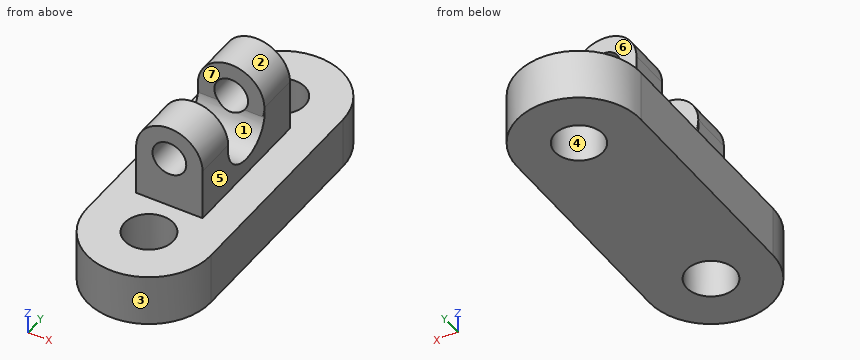
from build123d import *

# Parameters (mm, degrees)
F0_W      = 32.9013951123
F0_H      = 70.9037855268
F1_DEPTH  = 25.4
F2_DEPTH  = 50.8
F3_R      = 14.9412695824
F4_DEPTH  = 76.2
F5_W      = 16.4506975561
F5_H      = 20.7484884761
F7_W      = 16.4506975561
F7_H      = 20.7484884761
F9_R      = 8.3599226064
F10_DEPTH = 508


with BuildPart() as f1:
    # F0 (on Top) → F1 (new body)
    with BuildSketch(Plane.XY):
        with BuildLine():
            Line((28.4018162638, 52.9936365783), (9.7189312353, 52.9936365783))
            ThreePointArc((9.7189312353, 52.9936365783), (-2.1936381236, 41.0810672195), (-14.1062074824, 52.9936365783))
            Line((-14.1062074824, 52.9936365783), (-32.7890925109, 52.9936365783))
            Line((-32.7890925109, 52.9936365783), (-32.7890925109, -54.1481785476))
            Line((-32.7890925109, -54.1481785476), (-14.2189597558, -54.1481785476))
            ThreePointArc((-14.2189597558, -54.1481785476), (-2.1936381236, -42.1228569154), (9.8316835087, -54.1481785476))
            Line((9.8316835087, -54.1481785476), (28.4018162638, -54.1481785476))
            Line((28.4018162638, -54.1481785476), (28.4018162638, 52.9936365783))
        make_face()
        with Locations((-4.080792889, 0.9530261159)):
            Rectangle(F0_W, F0_H, mode=Mode.SUBTRACT)
        with BuildLine():
            ThreePointArc((-14.1062074824, 52.9936365783), (-2.1936381236, 64.9062059372), (9.7189312353, 52.9936365783))
            Line((9.7189312353, 52.9936365783), (28.4018162638, 52.9936365783))
            ThreePointArc((28.4018162638, 52.9936365783), (-2.1936381236, 83.5890909657), (-32.7890925109, 52.9936365783))
            Line((-32.7890925109, 52.9936365783), (-14.1062074824, 52.9936365783))
        make_face()
        with BuildLine():
            ThreePointArc((-32.7890925109, -54.1481785476), (-2.1936381236, -84.743632935), (28.4018162638, -54.1481785476))
            Line((28.4018162638, -54.1481785476), (9.8316835087, -54.1481785476))
            ThreePointArc((9.8316835087, -54.1481785476), (-2.1936381236, -66.1735001799), (-14.2189597558, -54.1481785476))
            Line((-14.2189597558, -54.1481785476), (-32.7890925109, -54.1481785476))
        make_face()
    extrude(amount=F1_DEPTH)

    # F0 (on Top) → F2 (join)
    with BuildSketch(Plane.XY):
        with Locations((-4.080792889, 0.9530261159)):
            Rectangle(F0_W, F0_H)
    extrude(amount=F2_DEPTH)

    # F3 (on face) → F4 (cut)
    with BuildSketch(Plane.YZ.offset(12.3699046671)):
        with Locations((0.9530261159, 48.1445454061)):
            Circle(F3_R)
    extrude(amount=-F4_DEPTH, mode=Mode.SUBTRACT)

    # F5 (on face) → F6 (revolve)
    with BuildSketch(Plane.XY.offset(50.8)):
        with Locations((4.1445558891, 26.0306746412)):
            Rectangle(F5_W, F5_H)
    revolve(axis=Axis((-4.080792889, 26.0306746412, 50.8), (0, -1, 0)))

    # F7 (on face) → F8 (revolve)
    with BuildSketch(Plane.XY.offset(50.8)):
        with Locations((-12.3061416671, -24.1246224094)):
            Rectangle(F7_W, F7_H)
    revolve(axis=Axis((-4.080792889, -24.1246224094, 50.8), (0, 1, 0)))

    # F9 (on face) → F10 (cut)
    with BuildSketch(Plane.XZ.offset(34.4988666475)):
        with Locations((-4.080792889, 50.8)):
            Circle(F9_R)
    extrude(amount=-F10_DEPTH, mode=Mode.SUBTRACT)


solid = f1.part
Read the model definition and answer for the solid it produces. Units are mm, in the model's axes. Face numbers are marked on the shaded views. A direction names the side the tool comes from. Give positions to 0.01 mm unless a question says otherwise; leave off trailing zeros. Write each loop counter-clockwise with the first axis right and the second up, starting at its lowest first coordinate (ties: lowest second). Pieces come first, ordered by that corner, then holes. Notation, with made-up numbers: (42, 60) - (80, 60) arc R23 cw to (80, 77) - close; hole circle Ø4 at (4.5, 25). An arc over 180 degrees is marked (long way). Use CSV: the item, a comma, the result in double quotes. Start each with the question number.
(1) Find section B-B (y = 22.5). Give the vertices of the cut face in (x, z).
(2) For the marked faces 5, 6 and 7, determine the directions among +Z, -Z, +X, -X, +Y, -Y from which every point of the face is accessible in a straight line to the end or side of a thin tool.
(3) Find section C-C (z = 56.5). Give the vertices of the cut face in (x, y).
(4) Find section D-D (y = 57). Give the vertices of the cut face in (x, z).
(5) Consider line 1 along Y through (x, z) = (-5, 8); line 2 along Z through (x, y) = (-13, -75); line 3 along X through (y, z) = (48.5, 12.5). Determine where each line is inside the solid, lowest interval first.
(6) Given P1, Ø2, axis at x = 5.5, z = 44, coming from the +Y side; P2, Ø10, axis at x = 12.5, y = -2.5, coming from the -Z side; P3, Ø1.5, axis at y = 20.5, z = 39.5, coming from the -X side; P4, Ø14.5, axis at x = -2.19, y = -54.15, coming from the -Z side, each flat-ended and moving along its own axis, determine where each tip first touches the part or whether it passes through.
(7) Determine the mould class of the marked faces 1, 2, 3 and 4 for opening direction Y: +Y half, -Y half, draft (parallel to the pull), parting line (faces both ways), or undercut.
Findings below:
1,outline,"(-32.79, 0) - (28.4, 0) - (28.4, 25.4) - (12.37, 25.4) - (12.37, 50.8) arc R16.45 ccw to (-20.53, 50.8) - (-20.53, 25.4) - (-32.79, 25.4) - close; hole circle Ø16.72 at (-4.08, 50.8)"
2,face 5,"+Z, +X, +Y, -Y"
2,face 6,"+Z, +X, -X, +Y"
2,face 7,"+Z, +X, -X"
3,outline,"(-19.51, -34.5) - (-10.2, -34.5) - (-10.2, -13.75) - (-19.51, -13.75) - close; (-19.51, 15.66) - (-10.2, 15.66) - (-10.2, 36.4) - (-19.51, 36.4) - close; (2.03, -34.5) - (11.35, -34.5) - (11.35, -13.75) - (2.03, -13.75) - close; (2.03, 15.66) - (11.35, 15.66) - (11.35, 36.4) - (2.03, 36.4) - close"
4,outline,"(-32.53, 0) - (-13.41, 0) - (-13.41, 25.4) - (-32.53, 25.4) - close; (9.03, 0) - (28.14, 0) - (28.14, 25.4) - (9.03, 25.4) - close"
5,line 1,"-84.61 to -65.84, -42.45 to 41.42, 64.57 to 83.46"
5,line 2,"0 to 25.4"
5,line 3,"-32.79 to -13.23, 8.84 to 28.4"
6,P1,"y = 36.4"
6,P2,"z = 0"
6,P3,"x = -20.53"
6,P4,"through"
7,face 1,"undercut"
7,face 2,"draft"
7,face 3,"-Y half"
7,face 4,"undercut"
